from build123d import *

# Parameters (mm, degrees)
F0_W      = 40
F0_H      = 43.4234265382
F1_DEPTH  = 2
F2_W      = 40
F2_H      = 43.4234265382
F2_W_2    = 36.8
F2_H_2    = 40.2234265382
F3_DEPTH  = 5
F5_DEPTH  = 1.6
F7_DEPTH  = 1
F8_DEPTH  = 4
F9_DEPTH  = 1
F11_DEPTH = 1.6
F13_DEPTH = 0.1


with BuildPart() as f1:
    # F0 (on Front) → F1 (new body)
    with BuildSketch(Plane.XZ):
        with Locations((-15.7519546337, 17.2915523872)):
            Rectangle(F0_W, F0_H)
    extrude(amount=F1_DEPTH)

    # F2 (on face) → F3 (join)
    with BuildSketch(Plane.XZ.offset(2)):
        with Locations((-15.7519546337, 17.2915523872)):
            Rectangle(F2_W, F2_H)
        with Locations((-15.7519546337, 17.2915523872)):
            Rectangle(F2_W_2, F2_H_2, mode=Mode.SUBTRACT)
    extrude(amount=F3_DEPTH)

    # F4 (on face) → F5 (cut, through all)
    with BuildSketch(Plane(origin=(0, 0, 37.4032656563), x_dir=(1, 0, 0), z_dir=(0, 0, -1))):
        with BuildLine():
            ThreePointArc((-4.8519546337, 4.5), (-4.1197215867, 2.732233047), (-2.3519546337, 2))
            ThreePointArc((-2.3519546337, 2), (-0.5841876808, 2.732233047), (0.1480453663, 4.5))
            ThreePointArc((0.1480453663, 4.5), (-0.5841876808, 6.267766953), (-2.3519546337, 7))
            ThreePointArc((-2.3519546337, 7), (-4.1197215867, 6.267766953), (-4.8519546337, 4.5))
        make_face()
        with BuildLine():
            ThreePointArc((-29.1519546337, 2), (-27.3841876808, 2.732233047), (-26.6519546337, 4.5))
            ThreePointArc((-26.6519546337, 4.5), (-27.3841876808, 6.267766953), (-29.1519546337, 7))
            ThreePointArc((-29.1519546337, 7), (-30.9197215867, 6.267766953), (-31.6519546337, 4.5))
            ThreePointArc((-31.6519546337, 4.5), (-30.9197215867, 2.732233047), (-29.1519546337, 2))
        make_face()
        with BuildLine():
            ThreePointArc((-29.1519546337, 7), (-27.3841876808, 6.267766953), (-26.6519546337, 4.5))
            Line((-26.6519546337, 4.5), (-26.6519546337, 7))
            Line((-26.6519546337, 7), (-29.1519546337, 7))
        make_face()
        with BuildLine():
            ThreePointArc((-31.6519546337, 4.5), (-30.9197215867, 6.267766953), (-29.1519546337, 7))
            Line((-29.1519546337, 7), (-31.6519546337, 7))
            Line((-31.6519546337, 7), (-31.6519546337, 4.5))
        make_face()
        with BuildLine():
            Line((-2.3519546337, 7), (-4.8519546337, 7))
            Line((-4.8519546337, 7), (-4.8519546337, 4.5))
            ThreePointArc((-4.8519546337, 4.5), (-4.1197215867, 6.267766953), (-2.3519546337, 7))
        make_face()
        with BuildLine():
            ThreePointArc((-2.3519546337, 7), (-0.5841876808, 6.267766953), (0.1480453663, 4.5))
            Line((0.1480453663, 4.5), (0.1480453663, 7))
            Line((0.1480453663, 7), (-2.3519546337, 7))
        make_face()
    extrude(amount=-F5_DEPTH, mode=Mode.SUBTRACT)

    # F6 (on face) → F7 (join)
    with BuildSketch(Plane.XZ.offset(2)):
        with BuildLine():
            Line((-17.2519546337, 25.3721127069), (-17.2519546337, 35.4344186057))
            ThreePointArc((-17.2519546337, 35.4344186057), (-21.0019546337, 30.4032656563), (-17.2519546337, 25.3721127069))
        make_face()
        with BuildLine():
            ThreePointArc((-14.2519546337, 25.3721127069), (-11.5425900736, 27.2657905568), (-10.5019546337, 30.4032656563))
            ThreePointArc((-10.5019546337, 30.4032656563), (-11.5425900736, 33.5407407558), (-14.2519546337, 35.4344186057))
            Line((-14.2519546337, 35.4344186057), (-14.2519546337, 25.3721127069))
        make_face()
    extrude(amount=F7_DEPTH)

    # F6 (on face) → F8 (join)
    with BuildSketch(Plane.XZ.offset(2)):
        with BuildLine():
            ThreePointArc((-14.2519546337, 35.4344186057), (-11.5425900736, 33.5407407558), (-10.5019546337, 30.4032656563))
            ThreePointArc((-10.5019546337, 30.4032656563), (-11.5425900736, 27.2657905568), (-14.2519546337, 25.3721127069))
            Line((-14.2519546337, 25.3721127069), (-14.2519546337, 24.3359351065))
            ThreePointArc((-14.2519546337, 24.3359351065), (-10.8306997125, 26.5505069044), (-9.5019546337, 30.4032656563))
            ThreePointArc((-9.5019546337, 30.4032656563), (-10.8306997125, 34.2560244081), (-14.2519546337, 36.470596206))
            Line((-14.2519546337, 36.470596206), (-14.2519546337, 35.4344186057))
        make_face()
        with BuildLine():
            ThreePointArc((-17.2519546337, 35.4344186057), (-15.7519546337, 35.6532656563), (-14.2519546337, 35.4344186057))
            Line((-14.2519546337, 35.4344186057), (-14.2519546337, 36.470596206))
            ThreePointArc((-14.2519546337, 36.470596206), (-15.7519546337, 36.6532656563), (-17.2519546337, 36.470596206))
            Line((-17.2519546337, 36.470596206), (-17.2519546337, 35.4344186057))
        make_face()
        with BuildLine():
            Line((-14.2519546337, 24.3359351065), (-14.2519546337, 25.3721127069))
            ThreePointArc((-14.2519546337, 25.3721127069), (-15.7519546337, 25.1532656563), (-17.2519546337, 25.3721127069))
            Line((-17.2519546337, 25.3721127069), (-17.2519546337, 24.3359351065))
            ThreePointArc((-17.2519546337, 24.3359351065), (-15.7519546337, 24.1532656563), (-14.2519546337, 24.3359351065))
        make_face()
        with BuildLine():
            ThreePointArc((-17.2519546337, 25.3721127069), (-21.0019546337, 30.4032656563), (-17.2519546337, 35.4344186057))
            Line((-17.2519546337, 35.4344186057), (-17.2519546337, 36.470596206))
            ThreePointArc((-17.2519546337, 36.470596206), (-22.0019546337, 30.4032656563), (-17.2519546337, 24.3359351065))
            Line((-17.2519546337, 24.3359351065), (-17.2519546337, 25.3721127069))
        make_face()
    extrude(amount=F8_DEPTH)

    # F6 (on face) → F9 (cut)
    with BuildSketch(Plane.XZ.offset(2)):
        with BuildLine():
            ThreePointArc((-17.2519546337, 35.4344186057), (-15.7519546337, 35.6532656563), (-14.2519546337, 35.4344186057))
            Line((-14.2519546337, 35.4344186057), (-14.2519546337, 36.470596206))
            ThreePointArc((-14.2519546337, 36.470596206), (-15.7519546337, 36.6532656563), (-17.2519546337, 36.470596206))
            Line((-17.2519546337, 36.470596206), (-17.2519546337, 35.4344186057))
        make_face()
        with BuildLine():
            Line((-14.2519546337, 24.3359351065), (-14.2519546337, 25.3721127069))
            ThreePointArc((-14.2519546337, 25.3721127069), (-15.7519546337, 25.1532656563), (-17.2519546337, 25.3721127069))
            Line((-17.2519546337, 25.3721127069), (-17.2519546337, 24.3359351065))
            ThreePointArc((-17.2519546337, 24.3359351065), (-15.7519546337, 24.1532656563), (-14.2519546337, 24.3359351065))
        make_face()
    extrude(amount=F9_DEPTH, mode=Mode.SUBTRACT)

    # F10 (on face) → F11 (cut, through all)
    with BuildSketch(Plane.XY.offset(-2.8201608819)):
        with BuildLine():
            Line((-13.2519546337, -7), (-13.2519546337, -4.5))
            ThreePointArc((-13.2519546337, -4.5), (-13.9841876808, -6.267766953), (-15.7519546337, -7))
            Line((-15.7519546337, -7), (-13.2519546337, -7))
        make_face()
        with BuildLine():
            ThreePointArc((-15.7519546337, -7), (-13.9841876808, -6.267766953), (-13.2519546337, -4.5))
            ThreePointArc((-13.2519546337, -4.5), (-13.984187679, -2.7322330488), (-15.7519546286, -2))
            ThreePointArc((-15.7519546286, -2), (-17.5197215849, -2.7322330452), (-18.2519546337, -4.5))
            ThreePointArc((-18.2519546337, -4.5), (-17.5197215867, -6.267766953), (-15.7519546337, -7))
        make_face()
        with BuildLine():
            Line((-18.2519546337, -7), (-15.7519546337, -7))
            ThreePointArc((-15.7519546337, -7), (-17.5197215867, -6.267766953), (-18.2519546337, -4.5))
            Line((-18.2519546337, -4.5), (-18.2519546337, -7))
        make_face()
    extrude(amount=-F11_DEPTH, mode=Mode.SUBTRACT)

    # F12 (on face) → F13 (cut)
    with BuildSketch(Plane.XZ.offset(2)):
        Polygon((-29.1519546337, 37.4032656563), (-33.1519546337, 37.4032656563), (-33.1519546337, 19.9032656563), (-25.1519546337, 19.9032656563), (-25.1519546337, 37.4032656563), align=None)
        Polygon((-2.3519546468, 37.4032656563), (-6.3519546337, 37.4032656563), (-6.3519546337, 19.9032656563), (1.6480453663, 19.9032656563), (1.6480453663, 37.4032656563), align=None)
        Polygon((-19.7519546337, 14.6798391181), (-19.7519546337, -2.8201608819), (-15.7519546337, -2.8201608819), (-11.7519546337, -2.8201608819), (-11.7519546337, 14.6798391181), align=None)
    extrude(amount=-F13_DEPTH, mode=Mode.SUBTRACT)


solid = f1.part
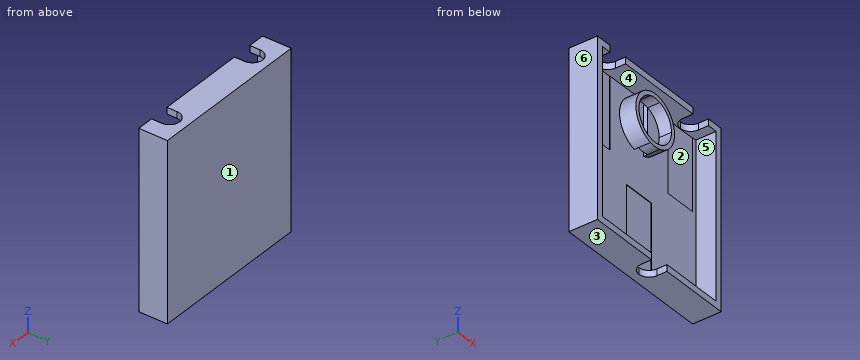
Geometry check sheet. Reference: the model listing, model coordinates, mm. Face numbers are marked on the shaded views. A direction names the side the tool comes from. Give positions to 0.01 mm unless a question says otherwise; leave off trailing zeros. Order: outer loops, then holes, each group sorted by start corner. A loop starts at its lowest first (then second) coordinate and runs counter-clockwise, first axis right, second up.
1. Sectioned sample at B-B (z = 18.5). Record the boundary of the cut face in (x, y), then the cut area to 3 significant figures.
Completed:
outline: (-35.75, -7) - (-34.15, -7) - (-34.15, -2) - (2.65, -2) - (2.65, -7) - (4.25, -7) - (4.25, 0) - (-35.75, 0) - close
area: 96.0 mm2
2. Access from +Z, -Z, +X, -X, +Y, -Y to the whole of each face (thin tool, end or side, straight path). Record for the marked faces 5 and 6.
Completed:
face 5: -Y
face 6: +Z, -Z, -X, +Y, -Y
3. Sectioned sample at C-C (x = -24.5). Record the boundary of the cut face in (y, z), then the cut area to 3 significant figures.
Completed:
outline: (-7, -4.42) - (0, -4.42) - (0, 39) - (-7, 39) - (-7, 37.4) - (-2, 37.4) - (-2, -2.82) - (-7, -2.82) - close
area: 103 mm2
4. Sectioned sample at D-D (y = -2.5). Record the boundary of the cut face in (x, z).
Completed:
outline: (-35.75, -4.42) - (-17.25, -4.42) - (-17.25, -2.82) - (-34.15, -2.82) - (-34.15, 37.4) - (-30.65, 37.4) - (-30.65, 39) - (-35.75, 39) - close; (-27.65, 37.4) - (-3.85, 37.4) - (-3.85, 39) - (-27.65, 39) - close; (-17.25, 24.34) - (-17.25, 36.47) arc R6.25 ccw to start; (-14.25, -4.42) - (4.25, -4.42) - (4.25, 39) - (-0.85, 39) - (-0.85, 37.4) - (2.65, 37.4) - (2.65, -2.82) - (-14.25, -2.82) - close; (-14.25, 24.34) arc R6.25 ccw to (-14.25, 36.47) - close
5. Depth check by flat-ended pin: pin 1 (1 mm diameter, centred on x = -28, z = 10, fed in from -Y); pin 2 (3 mm diameter, centred on x = -16, z = 24, fed in from -Y); pin 3 (1.1 mm diameter, centred on x = -18, z = 29, fed in from -Y). Enter the tip coordinate at first touch or a pass-through.
Completed:
pin 1: stops at y = -2
pin 2: stops at y = -6
pin 3: stops at y = -3
6. Scan lines: line 1 (X direction, y = -5.5, z = 8); line 2 (Z direction, x = -5, y = -4.75); line 3 (Y direction, x = -4.5, z = 20). Record each from-to range of solid material in increasing order.
Completed:
line 1: x = -35.75 to -34.15, 2.65 to 4.25
line 2: z = -4.42 to -2.82, 37.4 to 39
line 3: y = -1.9 to 0
7. Sectioned sample at A-A (y = -5.5). Record the boundary of the cut face in (x, z).
Completed:
outline: (-35.75, -4.42) - (-18.25, -4.42) - (-18.25, -2.82) - (-34.15, -2.82) - (-34.15, 37.4) - (-31.65, 37.4) - (-31.65, 39) - (-35.75, 39) - close; (-26.65, 37.4) - (-4.85, 37.4) - (-4.85, 39) - (-26.65, 39) - close; circle Ø12.5 at (-15.75, 30.4); (-13.25, -4.42) - (4.25, -4.42) - (4.25, 39) - (0.15, 39) - (0.15, 37.4) - (2.65, 37.4) - (2.65, -2.82) - (-13.25, -2.82) - close; hole circle Ø10.5 at (-15.75, 30.4)
8. Draft check along Z on the marked faces 1, 2, 3 and 4. Enter one of: pulls with the +Z half, pulls with the -Z half, needs draft (parallel to the pull), parting line crosses it, or undercut.
Completed:
face 1: needs draft
face 2: undercut
face 3: pulls with the -Z half
face 4: undercut
